Read the model definition and answer for the solid it produces. Units are mm, in the model's axes. A direction names the side the tool comes from. Coordinates: 2 decimals unless noted, no trailing zeros. Order: outer loops, then holes, each group sorted by start corner. A loop starts at its lowest first (then second) coordinate and runs counter-clockwise, first axis right, second up. Notation, with made-up numbers: M 47.25,79 L 98.25,79 A7 cw 98.25,84 Z; hole C 72.5,20 d9. An arc over 180 degrees is marked long. Use a Markdown table: item, result. Add a question column.
1) Find the intervals of material crossed by probe 1 along X at (y, z) = (250, 0.4) (3 decimals); probe 2 along Y at (x, z) = (49.05, 12.5) (3 decimals); probe 3 along X at (y, z) = (58, 22.5), in increasing order. Write a range as [from, to].
2) For faces 1 (the face through (25, 507, 1.5)), 2 (the face through (0, 493, 14)), determine the directions among +Z, -Z, +X, -X, +Y, -Y from which every point of the face is accessible in a straight line to the end or side of a thin tool.
3) Find section A-A on z = 18.75. Write down the section's boundary in (x, y).
4) Find section C-C on y = 824. Write down the section's boundary in (x, z), plus the area to 3 significant figures.
5) This flat-tipped pin is pushed along its axis until it touches: pin 1 Ø3 at (x, y) = (9, 443.5) entering from +Z. Where does it stop, or does it pass through?
6) Find section B-B on x = 25. Write down the section's boundary in (y, z), plus the area to 3 significant figures.
7) The mould has two halves that part along X. Classify faces 3 (the face through (25, 0, 1)), 4 (the face through (25, 972, 1)), 5 (the face through (1.5, 493, 14)), 6 (the face through (50, 507, 14)): released by +X, released by -X, zero draft, split by the parting line, or undercut.
Autodesk Inventor part; units mm, degrees
ref_plane "YZ Plane" through (0, 0, 0) normal (1, 0, 0) x (0, 1, 0)
ref_plane "XZ Plane" through (0, 0, 0) normal (0, 1, 0) x (-1, 0, 0)
ref_plane "XY Plane" through (0, 0, 0) normal (0, 0, 1) x (1, 0, 0)
sketch "Sketch1" plane through (0, 0, 0) normal (0, 0, 1) x (1, 0, 0)
  line L0 (0, 0) -> (50, 0)
  line L1 (50, 0) -> (50, 1000)
  line L2 (50, 1000) -> (0, 1000)
  line L3 (0, 1000) -> (0, 0)
  dimension "d0" = 50
  dimension "d1" = 1000
extrude "Plate1" add sketch "Sketch1" along normal blind 1.5
sketch "Sketch2" plane through (48.5, 1000, 0) normal (1, 0, 0) x (0, 1, 0)
  line L0 (-1000, 0) -> (0, 0)
  line L1 (0, 0) -> (0, 25)
  line L2 (0, 25) -> (-1000, 25)
  line L3 (-1000, 25) -> (-1000, 0)
edge flange "Flange1" height 20 angle 90 thickness 1.5 bend radius 1.5 thickness toward (1, 0, 0) relief tear relief width 1.5 relief depth 0.75 edges at (50, 500, 1.5) wall of the first edge with corners at (48.5, 0, 0) (48.5, 1000, 0) (48.5, 1000, 25) (48.5, 0, 25)
bend "Bend1"
corner "Corner1"
sketch "Sketch3" plane through (1.5, 0, 0) normal (-1, 0, 0) x (0, -1, 0)
  line L0 (-1000, 0) -> (0, 0)
  line L1 (0, 0) -> (0, 25)
  line L2 (0, 25) -> (-1000, 25)
  line L3 (-1000, 25) -> (-1000, 0)
edge flange "Flange2" height 20 angle 90 thickness 1.5 bend radius 1.5 thickness toward (-1, 0, 0) relief tear relief width 1.5 relief depth 0.75 edges at (0, 500, 1.5) wall of the first edge with corners at (1.5, 1000, 0) (1.5, 0, 0) (1.5, 0, 25) (1.5, 1000, 25)
bend "Bend2"
corner "Corner2"
sketch "Sketch4" plane through (0, 0, 25) normal (-1, 0, 0) x (0, 0, 1)
  circle A0 centre (-12.5, 125) radius 1.675
  line L0 (0, 0) -> (-22, 0)
  circle A1 centre (-12.5, 375) radius 1.675
  line L1 (-22, 1000) -> (-22, 0)
  circle A2 centre (-12.5, 625) radius 1.675
  circle A3 centre (-12.5, 875) radius 1.675
  line L2 (-22, 1000) -> (0, 1000)
  line L3 (-25, 1000) -> (-25, 0)
  dimension "d23" = 3.35
  dimension "d24" = 125
  dimension "d25" = 3.35
  dimension "d26" = 250
  dimension "d29" = 3.35
  dimension "d30" = 250
  dimension "d32" = 3.35
  dimension "d33" = 250
  dimension "d35" = 125
  dimension "d56" = 10
  dimension "d57" = 10
  dimension "d58" = 10
  dimension "d59" = 10
hole "Hole1" at (0, 375, 12.5) at (0, 625, 12.5) at (0, 125, 12.5) at (0, 875, 12.5) direction (1, 0, 0) diameter 3.35 end through all
sketch "Sketch5" plane through (0, 0, 0) normal (0, 0, -1) x (-1, 0, 0)
  circle A0 centre (-25, 20) radius 8
  line L0 (-3, 0) -> (-47, 0)
  line L1 (0, 1000) -> (0, 0)
  circle A1 centre (-25, 980) radius 8
  line L2 (-47, 1000) -> (-3, 1000)
  dimension "d43" = 16
  dimension "d44" = 20
  dimension "d45" = 25
  dimension "d53" = 16
  dimension "d54" = 20
  dimension "d55" = 25
hole "Hole2" at (25, 20, 0) at (25, 980, 0) direction (0, 0, 1) diameter 16 end through all
sketch "Sketch6" plane through (0, 0, 0) normal (0, 0, -1) x (-1, 0, 0)
  circle A0 centre (-37.5, 125) radius 1.675
  line L0 (-3, 0) -> (-47, 0)
  line L1 (-50, 0) -> (-50, 1000)
  circle A1 centre (-12.5, 125) radius 1.675
  circle A2 centre (-37.5, 250) radius 1.675
  circle A3 centre (-12.5, 250) radius 1.675
  circle A4 centre (-37.5, 375) radius 1.675
  circle A5 centre (-12.5, 375) radius 1.675
  circle A6 centre (-37.5, 500) radius 1.675
  circle A7 centre (-12.5, 500) radius 1.675
  circle A8 centre (-37.5, 625) radius 1.675
  circle A9 centre (-12.5, 625) radius 1.675
  circle A10 centre (-37.5, 750) radius 1.675
  circle A11 centre (-12.5, 750) radius 1.675
  circle A12 centre (-37.5, 875) radius 1.675
  circle A13 centre (-12.5, 875) radius 1.675
  point P0 (0, 0)
  dimension "d60" = 3.35
  dimension "d61" = 125
  dimension "d62" = 12.5
  dimension "d63" = 3.35
  dimension "d64" = 25
  dimension "d67" = 125
extrude "Cut1" cut sketch "Sketch6" against normal blind 1.5
sketch "Sketch7" plane through (0, 0, 25) normal (-1, 0, 0) x (0, 0, 1)
  point P0 (-25, 0)
equation "\"d0\" = A_height"
equation "\"d1\" = A_length"
equation "\"d23\" = rivet_diameter"
equation "\"d24\" = 0.5 * rivet_displacement"
equation "\"d25\" = rivet_diameter"
equation "\"d26\" = rivet_displacement"
equation "\"d29\" = rivet_diameter"
equation "\"d30\" = rivet_displacement"
equation "\"d32\" = rivet_diameter"
equation "\"d33\" = rivet_displacement"
equation "\"d56\" = 0.25 * A_width"
equation "\"d57\" = 0.25 * A_width"
equation "\"d58\" = 0.25 * A_width"
equation "\"d59\" = 0.25 * A_width"
equation "\"d36\" = rivet_diameter"
equation "\"d41\" = Thickness"
equation "\"d43\" = A_joint_diameter"
equation "\"d45\" = 0.5 * A_height"
equation "\"d53\" = A_joint_diameter"
equation "\"d55\" = 0.5 * A_height"
equation "\"d46\" = A_joint_diameter"
equation "\"d51\" = Thickness"
equation "\"d60\" = rivet_diameter"
equation "\"d61\" = 0.5 * rivet_displacement"
equation "\"d63\" = rivet_diameter"
equation "\"d67\" = 0.5 * rivet_displacement"
equation "\"d72\" = Thickness"
equation "\"d2\" = Thickness"
equation "\"d3\" = BendReliefWidth"
equation "\"d4\" = BendReliefDepth"
equation "\"d5\" = MinimumRemnant"
equation "\"d6\" = TransitionRadius"
equation "\"d7\" = 0.5 * A_width"
equation "\"d9\" = BendRadius"
equation "\"d10\" = CornerReliefSize"
equation "\"d11\" = GapSize"
equation "\"d12\" = JacobiRadiusSize"
equation "\"d13\" = BendReliefWidth"
equation "\"d14\" = BendReliefDepth"
equation "\"d15\" = MinimumRemnant"
equation "\"d16\" = TransitionRadius"
equation "\"d17\" = 0.5 * A_width"
equation "\"d19\" = BendRadius"
equation "\"d20\" = CornerReliefSize"
equation "\"d21\" = GapSize"
equation "\"d22\" = JacobiRadiusSize"
equation "\"Thickness\" = plate_thickness"
equation "\"BendRadius\" = Thickness"
equation "\"BendReliefWidth\" = Thickness"
equation "\"BendReliefDepth\" = 0.5 * Thickness"
equation "\"CornerReliefSize\" = 4 * Thickness"
equation "\"MinimumRemnant\" = 2 * Thickness"
equation "\"TransitionRadius\" = BendRadius"
equation "\"JacobiRadiusSize\" = BendRadius"
equation "\"GapSize\" = Thickness"
equation "\"A_length\" = 1000"
equation "\"l___________\" = 0"
equation "\"l__________\" = 0"
equation "\"l_________\" = 0"
equation "\"rivet_diameter\" = 3.35"
equation "\"rivet_displacement\" = 250"
equation "\"l________\" = 0"
equation "\"plate_thickness\" = 1.5"
equation "\"A_joint_diameter\" = 16"
equation "\"A_height\" = 50"
equation "\"A_joint_tolerance\" = 3"
equation "\"A_B_spacing\" = 2"
equation "\"L_Piston_Bottom\" = 21"
equation "\"L_Piston_Top\" = 25"
properties part number "Beam_A1"
Check result:
| question | item | result |
|---|---|---|
| 1 | probe 1 | x = [1.503, 10.825], [14.175, 35.825], [39.175, 48.497] |
| 1 | probe 2 | y = [0, 123.325], [126.675, 373.325], [376.675, 623.325], [626.675, 873.325], [876.675, 1000] |
| 1 | probe 3 | x = [0, 1.5], [48.5, 50] |
| 2 | face 1 | +Z, +Y, -Y |
| 2 | face 2 | +Z, -Z, -X, +Y, -Y |
| 3 | outline | M 0,0 L 1.5,0 L 1.5,1000 L 0,1000 Z; M 48.5,0 L 50,0 L 50,1000 L 48.5,1000 Z |
| 4 | outline | M 0,3 A3 ccw 3,0 L 47,0 A3 ccw 50,3 L 50,25 L 48.5,25 L 48.5,3 A1.5 cw 47,1.5 L 3,1.5 A1.5 cw 1.5,3 L 1.5,25 L 0,25 Z |
| 4 | area | 143 mm2 |
| 5 | pin 1 | stops at z = 1.5 |
| 6 | outline | M 0,0 L 12,0 L 12,1.5 L 0,1.5 Z; M 28,0 L 972,0 L 972,1.5 L 28,1.5 Z; M 988,0 L 1000,0 L 1000,1.5 L 988,1.5 Z |
| 6 | area | 1,450 mm2 |
| 7 | face 3 | zero draft |
| 7 | face 4 | undercut |
| 7 | face 5 | undercut |
| 7 | face 6 | released by +X |
